Build history of the part. All positions in model axes, mm. A direction names the side the tool comes from. Coordinates: 2 decimals unless noted, no trailing zeros. Order: outer loops, then holes, each group sorted by start corner. A loop starts at its lowest first (then second) coordinate and runs counter-clockwise, first axis right, second up. Notation, with made-up numbers: M -15.75,-32.75 L 32.25,-32.75 A8 cw 32.25,-18.75 Z; hole C 79,76.25 d3. An arc over 180 degrees is marked long. Write item = value, one per line. Start each with the question number.
Q1. Drill centre lines: probe 1 along Z at (x, y) = (20, -4.5); probe 2 along Z at (x, y) = (180, -1.85); probe 3 along Z at (x, y) = (170, -3.75). Where is each one in solid material? Low to high.
Q2. Pull direction Z, two halves, no side cores. Call faces 4 (the face through (159, -3, -4)), 5 (the face through (159.7, -3, 85)), 6 (the face through (76, -6, 62)), 7 (the face through (20, -3, 122)): released by +Z, released by -Z, zero draft, split by the parting line, or undercut.
Q3. Band-saw the part on D-D on y = -2.7. Write the cut outline in (x, z) (3 decimals), plus the area to 3 significant figures.
Q4. Band-saw the part on C-C on z = 110. Write the cut outline in (x, y), plus the area to 3 significant figures.
Q5. Band-saw the part on A-A on x = 20. Write the cut outline in (y, z).
Q6. Pin check, flat tips, straight feed: P1, Ø3, axis at x = 171, y = -2.5, coming from the +Z side; P2, Ø13, axis at x = 61.03, z = 87.5, coming from the +Y side; P3, Ø1.5, axis at x = 49, y = -5, coming from the -Z side; P4, Ø6, axis at x = 138.97, z = 42.5, coming from the -Y side. Stop position of each tip, or through.
Q7. Band-saw the part on B-B on x = 125.5. Write the cut outline in (y, z), plus the area to 3 significant figures.
Q8. 3-axis set-ups, long thin cutter, end or side, ignore diameter. For faces 1 (the face through (41, -3, -4)), 2 (the face through (18.92, -2.96, 105.12)), 3 (the face through (180, -3, 90.3)): which of +Z, -Z, +X, -X, +Y, -Y reach the whole face in a straight line?
```python
from build123d import *

# Parameters (mm, degrees)
F0_R     = 5
F0_W     = 40
F0_H     = 8
F1_DEPTH = 6


# Not quite as in the source:
# - a feature names something its author has since deleted; it is built from what else it names


with BuildPart() as f1:
    # F0 (on Front) → F1 (new body)
    with BuildSketch(Plane.XZ):
        with BuildLine():
            Line((0, 122), (0, 0))
            Line((0, 0), (40, 0))
            Line((40, 0), (42, 0))
            Line((42, 0), (158, 0))
            Line((158, 0), (160, 0))
            Line((160, 0), (200, 0))
            Line((200, 0), (200, 39.7))
            Line((200, 39.7), (159.7, 39.7))
            Line((159.7, 39.7), (159.7, 49.85))
            Line((159.7, 49.85), (126.2405697347, 49.85))
            Line((126.2405697347, 49.85), (100, 49.85))
            ThreePointArc((100, 49.85), (86.8797151327, 57.425), (86.8797151327, 72.575))
            ThreePointArc((86.8797151327, 72.575), (92.425, 78.1202848673), (100, 80.15))
            Line((100, 80.15), (159.7, 80.15))
            Line((159.7, 80.15), (159.7, 90.3))
            Line((159.7, 90.3), (200, 90.3))
            Line((200, 90.3), (200, 122))
            Line((200, 122), (160, 122))
            Line((160, 122), (158, 130))
            Line((158, 130), (42, 130))
            Line((42, 130), (40, 122))
            Line((40, 122), (0, 122))
        make_face()
        with Locations((20, 20)):
            Circle(F0_R, mode=Mode.SUBTRACT)
        with Locations((180, 20)):
            Circle(F0_R, mode=Mode.SUBTRACT)
        with BuildLine():
            ThreePointArc((143.9711431703, 42.5), (137.6770479448, 37.6703708686), (134.6410161514, 45))
            ThreePointArc((134.6410161514, 45), (140.2652383958, 47.3296291314), (143.9711431703, 42.5))
        make_face(mode=Mode.SUBTRACT)
        with BuildLine():
            ThreePointArc((66.0288568297, 87.5), (65.8584859611, 86.2059047745), (65.3589838486, 85))
            ThreePointArc((65.3589838486, 85), (56.1992276983, 88.7940952255), (66.0288568297, 87.5))
        make_face(mode=Mode.SUBTRACT)
        with Locations((20, 110)):
            Circle(F0_R, mode=Mode.SUBTRACT)
        with Locations((180, 110)):
            Circle(F0_R, mode=Mode.SUBTRACT)
        with Locations((20, -4)):
            Rectangle(F0_W, F0_H)
        with Locations((180, -4)):
            Rectangle(F0_W, F0_H)
        Polygon((42, 0), (40, 0), (40, -8), align=None)
        Polygon((160, 0), (158, 0), (160, -8), align=None)
    extrude(amount=F1_DEPTH)


solid = f1.part
```
Recorded:
q1.probe_1 = -8 to 15, 25 to 105, 115 to 122
q1.probe_2 = -8 to 15, 25 to 39.7, 90.3 to 105, 115 to 122
q1.probe_3 = -8 to 39.7, 90.3 to 122
q2.face_4 = released by -Z
q2.face_5 = undercut
q2.face_6 = zero draft
q2.face_7 = released by +Z
q3.outline = M 0,-8 L 40,-8 L 42,0 L 158,0 L 160,-8 L 200,-8 L 200,39.7 L 159.7,39.7 L 159.7,49.85 L 100,49.85 A15.15 cw 100,80.15 L 159.7,80.15 L 159.7,90.3 L 200,90.3 L 200,122 L 160,122 L 158,130 L 42,130 L 40,122 L 0,122 Z; hole C 20,20 d10; hole C 20,110 d10; hole C 61.029,87.5 d10; hole C 138.971,42.5 d10; hole C 180,20 d10; hole C 180,110 d10
q3.area = 21,300 mm2
q4.outline = M 0,-6 L 15,-6 L 15,0 L 0,0 Z; M 25,-6 L 175,-6 L 175,0 L 25,0 Z; M 185,-6 L 200,-6 L 200,0 L 185,0 Z
q4.area = 1,080 mm2
q5.outline = M -6,-8 L 0,-8 L 0,15 L -6,15 Z; M -6,25 L 0,25 L 0,105 L -6,105 Z; M -6,115 L 0,115 L 0,122 L -6,122 Z
q6.P1 = 122
q6.P2 = 0
q6.P3 = 0
q6.P4 = through
q7.outline = M -6,0 L 0,0 L 0,49.85 L -6,49.85 Z; M -6,80.15 L 0,80.15 L 0,130 L -6,130 Z
q7.area = 598 mm2
q8.face_1 = -Z, +Y, -Y
q8.face_2 = +Y, -Y
q8.face_3 = +X, +Y, -Y
